Input: dimensioned drawing with shaded views. Units: mm. Origin: part minimum x, y, z. A direction names the side the tool comes from. Give positions to 0.01 mm unless a question says otherwise; leave off trailing zeros. Loops run counter-clockwise (first coordinate to the right, second up) from the corner with the lowest first, then second, coordinate; pieces in that order, holes last. Notation, with made-up numbers: M 43.5,-20 L 71.5,-20 A16 cw 71.5,5 Z; hole C 85.25,19.25 d8. An arc over 180 degrees is marked long. One line per question, with ' | ' between items. Start each with the question number.
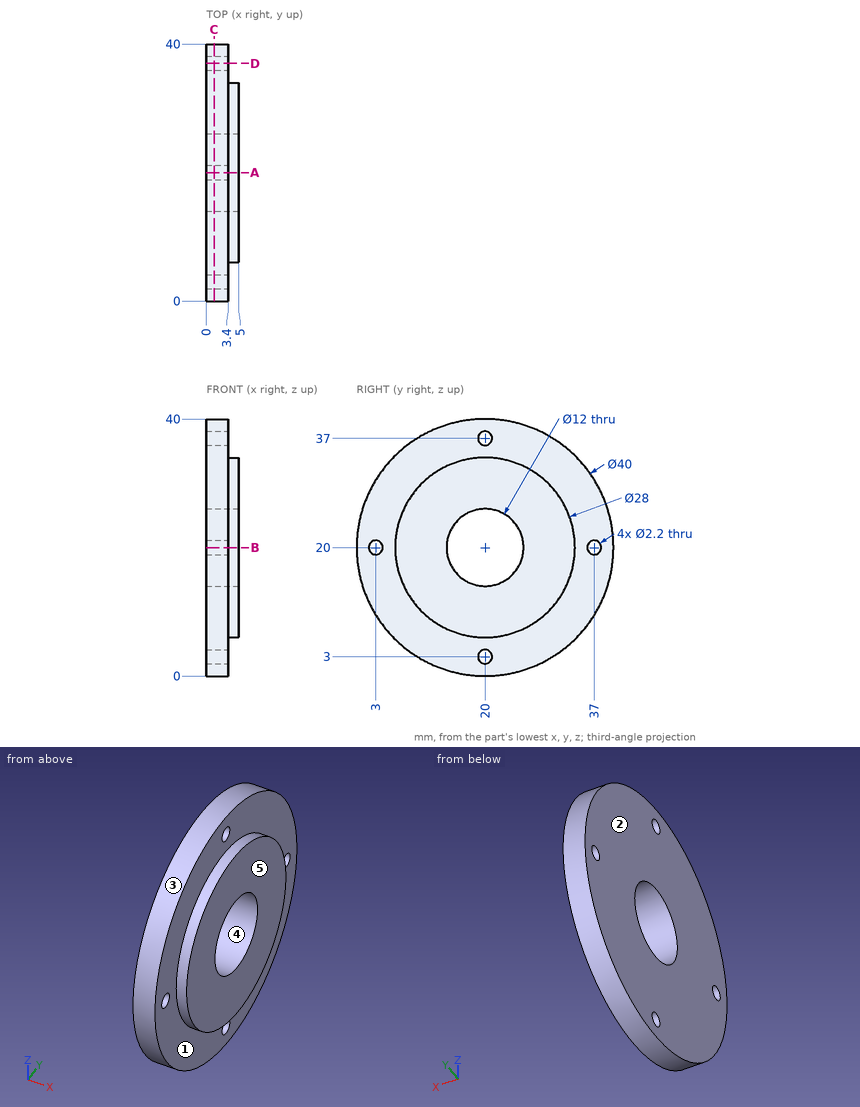
Q1. Set-up query: the marked faces 1 and 2. Return all of +Z, -Z, +X, -X, +Y, -Y with unobstructed straight access to the full face (end or side cutting, diameter ignored); none if empty.
Q2. Section A-A, the plane y = 20. Output: boundary loops of the cut face in (x, z).
Q3. Section C-C, the plane x = 1.2. Output: boundary loops of the cut face in (y, z), plus the area to 3 significant figures.
Q4. Material intervals for L1, parallel to X at y = 31.5, z = 4; L2, parallel to Z at x = 1, y = 20.5; L3, parallel to Z at x = 1, y = 3, sorted ascending.
Q5. Contact query for flat-ended pins moving along their axis: pin 1 (2 mm diameter, centred on x = 3, z = 13, fed in from +Y); pin 2 (1.3 mm diameter, centred on y = 3, z = 20, fed in from +X); pin 3 (3 mm diameter, centred on y = 32.5, z = 4.5, fed in from +X); pin 4 (1.5 mm diameter, centred on x = 1, z = 32, fed in from -Y). Output: stop coordinate, or through.
Q6. Draft query along Y for the marked faces 3, 4 and 5. Return one class per face: released by +Y, released by -Y, zero draft, split by the parting line, or undercut.
Q7. Section D-D, the plane y = 37. Output: boundary loops of the cut face in (x, z).
Model answer:
1) face 1: +X | face 2: +Z, -Z, -X, +Y, -Y
2) outline: M 0,0 L 3.4,0 L 3.4,1.9 L 0,1.9 Z; M 0,4.1 L 3.4,4.1 L 3.4,6 L 5,6 L 5,14 L 0,14 Z; M 0,26 L 5,26 L 5,34 L 3.4,34 L 3.4,35.9 L 0,35.9 Z; M 0,38.1 L 3.4,38.1 L 3.4,40 L 0,40 Z
3) outline: C 20,20 d40; hole C 3,20 d2.2; hole C 20,20 d12; hole C 20,3 d2.2; hole C 20,37 d2.2; hole C 37,20 d2.2 | area: 1,130 mm^2
4) L1: x = 0 to 3.4 | L2: z = 0.01 to 2.02, 3.98 to 14.02, 25.98 to 36.02, 37.98 to 39.99 | L3: z = 9.46 to 18.9, 21.1 to 30.54
5) pin 1: stops at y = 39.08 | pin 2: passes through | pin 3: stops at x = 3.4 | pin 4: stops at y = 3.46
6) face 3: split by the parting line | face 4: undercut | face 5: zero draft
7) outline: M 0,9.46 L 3.4,9.46 L 3.4,18.9 L 0,18.9 Z; M 0,21.1 L 3.4,21.1 L 3.4,30.54 L 0,30.54 Z
